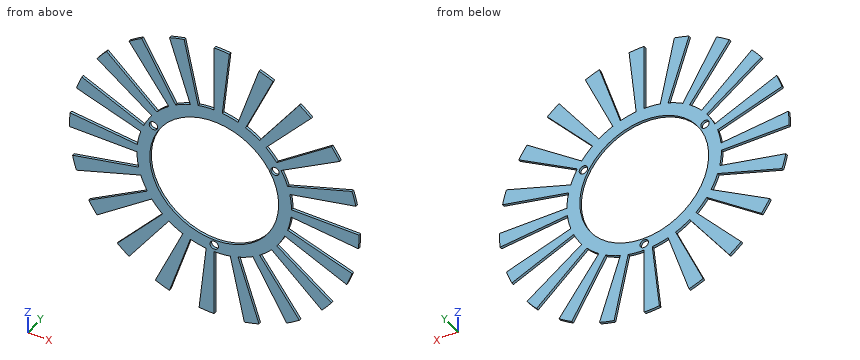
```python
from build123d import *

# Parameters (mm, degrees)
SKETCH1_R           = 30.25
SKETCH1_R_2         = 25.25
EXTRUDE_THIN1_DEPTH = 1
SKETCH2_R           = 1.65
CUT_EXTRUDE3_DEPTH  = 10
BOSS_EXTRUDE1_DEPTH = 1


with BuildPart() as part:
    # Sketch1 → Extrude-Thin1 (new body)
    with BuildSketch(Plane(origin=(0, 0, 0), x_dir=(1, 0, 0), z_dir=(0, 1, 0))):
        Circle(SKETCH1_R)
        Circle(SKETCH1_R_2, mode=Mode.SUBTRACT)
    extrude(amount=-EXTRUDE_THIN1_DEPTH)

    # Sketch2 → Cut-Extrude3 (cut)
    with BuildSketch(Plane(origin=(0, 0, 0), x_dir=(1, 0, 0), z_dir=(0, 1, 0))):
        with Locations((0, 27.5)):
            Circle(SKETCH2_R)
        with Locations((23.815698604, -13.75)):
            Circle(SKETCH2_R)
        with Locations((-23.815698604, -13.75)):
            Circle(SKETCH2_R)
    extrude(amount=-CUT_EXTRUDE3_DEPTH, mode=Mode.SUBTRACT)

    # Sketch5 → Boss-Extrude1 (add)
    with BuildSketch(Plane.XZ.offset(1)):
        with BuildLine():
            Line((0, 56.75), (0, 30.25))
            ThreePointArc((0, 30.25), (1.583162676, 30.208543426), (3.161986014, 30.084287335))
            Line((3.161986014, 30.084287335), (5.93199029, 56.439117562))
            ThreePointArc((5.93199029, 56.439117562), (2.970065517, 56.672226097), (0, 56.75))
        make_face()
        with BuildLine():
            Line((17.536714431, 53.9724573), (9.34776408, 28.769459618))
            ThreePointArc((9.34776408, 28.769459618), (10.840630474, 28.240807902), (12.303783453, 27.634750094))
            Line((12.303783453, 27.634750094), (23.082304495, 51.843704721))
            ThreePointArc((23.082304495, 51.843704721), (20.337381137, 52.980689204), (17.536714431, 53.9724573))
        make_face()
        with BuildLine():
            Line((33.356813068, 45.911714431), (17.780503882, 24.47276408))
            ThreePointArc((17.780503882, 24.47276408), (19.036941829, 23.508665334), (20.241200842, 22.480130971))
            Line((20.241200842, 22.480130971), (37.973161911, 42.173468846))
            ThreePointArc((37.973161911, 42.173468846), (35.713932192, 44.103033313), (33.356813068, 45.911714431))
        make_face()
        with BuildLine():
            Line((45.911714431, 33.356813068), (24.47276408, 17.780503882))
            ThreePointArc((24.47276408, 17.780503882), (25.36978468, 16.475330809), (26.197268464, 15.125))
            Line((26.197268464, 15.125), (49.146941665, 28.375))
            ThreePointArc((49.146941665, 28.375), (47.594554731, 30.908265237), (45.911714431, 33.356813068))
        make_face()
        with BuildLine():
            Line((53.9724573, 17.536714431), (28.769459618, 9.34776408))
            ThreePointArc((28.769459618, 9.34776408), (29.219256245, 7.829276114), (29.588964922, 6.289328647))
            Line((29.588964922, 6.289328647), (55.509876342, 11.798988454))
            ThreePointArc((55.509876342, 11.798988454), (54.816290642, 14.68798081), (53.9724573, 17.536714431))
        make_face()
        with BuildLine():
            Line((56.75, 0), (30.25, 0))
            ThreePointArc((30.25, 0), (30.208543426, -1.583162676), (30.084287335, -3.161986014))
            Line((30.084287335, -3.161986014), (56.439117562, -5.93199029))
            ThreePointArc((56.439117562, -5.93199029), (56.672226097, -2.970065517), (56.75, 0))
        make_face()
        with BuildLine():
            Line((53.9724573, -17.536714431), (28.769459618, -9.34776408))
            ThreePointArc((28.769459618, -9.34776408), (28.240807902, -10.840630474), (27.634750094, -12.303783453))
            Line((27.634750094, -12.303783453), (51.843704721, -23.082304495))
            ThreePointArc((51.843704721, -23.082304495), (52.980689204, -20.337381137), (53.9724573, -17.536714431))
        make_face()
        with BuildLine():
            Line((45.911714431, -33.356813068), (24.47276408, -17.780503882))
            ThreePointArc((24.47276408, -17.780503882), (23.508665334, -19.036941829), (22.480130971, -20.241200842))
            Line((22.480130971, -20.241200842), (42.173468846, -37.973161911))
            ThreePointArc((42.173468846, -37.973161911), (44.103033313, -35.713932192), (45.911714431, -33.356813068))
        make_face()
        with BuildLine():
            Line((33.356813068, -45.911714431), (17.780503882, -24.47276408))
            ThreePointArc((17.780503882, -24.47276408), (16.475330809, -25.36978468), (15.125, -26.197268464))
            Line((15.125, -26.197268464), (28.375, -49.146941665))
            ThreePointArc((28.375, -49.146941665), (30.908265237, -47.594554731), (33.356813068, -45.911714431))
        make_face()
        with BuildLine():
            Line((17.536714431, -53.9724573), (9.34776408, -28.769459618))
            ThreePointArc((9.34776408, -28.769459618), (7.829276114, -29.219256245), (6.289328647, -29.588964922))
            Line((6.289328647, -29.588964922), (11.798988454, -55.509876342))
            ThreePointArc((11.798988454, -55.509876342), (14.68798081, -54.816290642), (17.536714431, -53.9724573))
        make_face()
        with BuildLine():
            Line((0, -56.75), (0, -30.25))
            ThreePointArc((0, -30.25), (-1.583162676, -30.208543426), (-3.161986014, -30.084287335))
            Line((-3.161986014, -30.084287335), (-5.93199029, -56.439117562))
            ThreePointArc((-5.93199029, -56.439117562), (-2.970065517, -56.672226097), (0, -56.75))
        make_face()
        with BuildLine():
            Line((-17.536714431, -53.9724573), (-9.34776408, -28.769459618))
            ThreePointArc((-9.34776408, -28.769459618), (-10.840630474, -28.240807902), (-12.303783453, -27.634750094))
            Line((-12.303783453, -27.634750094), (-23.082304495, -51.843704721))
            ThreePointArc((-23.082304495, -51.843704721), (-20.337381137, -52.980689204), (-17.536714431, -53.9724573))
        make_face()
        with BuildLine():
            Line((-33.356813068, -45.911714431), (-17.780503882, -24.47276408))
            ThreePointArc((-17.780503882, -24.47276408), (-19.036941829, -23.508665334), (-20.241200842, -22.480130971))
            Line((-20.241200842, -22.480130971), (-37.973161911, -42.173468846))
            ThreePointArc((-37.973161911, -42.173468846), (-35.713932192, -44.103033313), (-33.356813068, -45.911714431))
        make_face()
        with BuildLine():
            Line((-45.911714431, -33.356813068), (-24.47276408, -17.780503882))
            ThreePointArc((-24.47276408, -17.780503882), (-25.36978468, -16.475330809), (-26.197268464, -15.125))
            Line((-26.197268464, -15.125), (-49.146941665, -28.375))
            ThreePointArc((-49.146941665, -28.375), (-47.594554731, -30.908265237), (-45.911714431, -33.356813068))
        make_face()
        with BuildLine():
            Line((-53.9724573, -17.536714431), (-28.769459618, -9.34776408))
            ThreePointArc((-28.769459618, -9.34776408), (-29.219256245, -7.829276114), (-29.588964922, -6.289328647))
            Line((-29.588964922, -6.289328647), (-55.509876342, -11.798988454))
            ThreePointArc((-55.509876342, -11.798988454), (-54.816290642, -14.68798081), (-53.9724573, -17.536714431))
        make_face()
        with BuildLine():
            Line((-56.75, 0), (-30.25, 0))
            ThreePointArc((-30.25, 0), (-30.208543426, 1.583162676), (-30.084287335, 3.161986014))
            Line((-30.084287335, 3.161986014), (-56.439117562, 5.93199029))
            ThreePointArc((-56.439117562, 5.93199029), (-56.672226097, 2.970065517), (-56.75, 0))
        make_face()
        with BuildLine():
            Line((-53.9724573, 17.536714431), (-28.769459618, 9.34776408))
            ThreePointArc((-28.769459618, 9.34776408), (-28.240807902, 10.840630474), (-27.634750094, 12.303783453))
            Line((-27.634750094, 12.303783453), (-51.843704721, 23.082304495))
            ThreePointArc((-51.843704721, 23.082304495), (-52.980689204, 20.337381137), (-53.9724573, 17.536714431))
        make_face()
        with BuildLine():
            Line((-45.911714431, 33.356813068), (-24.47276408, 17.780503882))
            ThreePointArc((-24.47276408, 17.780503882), (-23.508665334, 19.036941829), (-22.480130971, 20.241200842))
            Line((-22.480130971, 20.241200842), (-42.173468846, 37.973161911))
            ThreePointArc((-42.173468846, 37.973161911), (-44.103033313, 35.713932192), (-45.911714431, 33.356813068))
        make_face()
        with BuildLine():
            Line((-33.356813068, 45.911714431), (-17.780503882, 24.47276408))
            ThreePointArc((-17.780503882, 24.47276408), (-16.475330809, 25.36978468), (-15.125, 26.197268464))
            Line((-15.125, 26.197268464), (-28.375, 49.146941665))
            ThreePointArc((-28.375, 49.146941665), (-30.908265237, 47.594554731), (-33.356813068, 45.911714431))
        make_face()
        with BuildLine():
            Line((-17.536714431, 53.9724573), (-9.34776408, 28.769459618))
            ThreePointArc((-9.34776408, 28.769459618), (-7.829276114, 29.219256245), (-6.289328647, 29.588964922))
            Line((-6.289328647, 29.588964922), (-11.798988454, 55.509876342))
            ThreePointArc((-11.798988454, 55.509876342), (-14.68798081, 54.816290642), (-17.536714431, 53.9724573))
        make_face()
    extrude(amount=-BOSS_EXTRUDE1_DEPTH)


solid = part.part
```
Work out the finished part from the listing and answer in its coordinate system (mm). Give positions to 0.01 mm unless a question says otherwise; leave off trailing zeros. Loops run counter-clockwise (first coordinate to the right, second up) from the corner with the lowest first, then second, coordinate; pieces in that order, holes last. Notation, with made-up numbers: (89.5, 4) -> (132.5, 4) arc R14 ccw to (132.5, 13) -> close; hole circle Ø1 at (-2, 78.25). An arc over 180 degrees is marked (long way). Use CSV: the item, a comma, the result in double quotes.
1. The part is cut by section A-A (z = 44.5). Write down the section's boundary in (x, y).
Found:
outline,"(-32.33, -1) -> (-25.69, -1) -> (-25.69, 0) -> (-32.33, 0) -> close; (-14.46, -1) -> (-9.46, -1) -> (-9.46, 0) -> (-14.46, 0) -> close; (0, -1) -> (4.68, -1) -> (4.68, 0) -> (0, 0) -> close; (14.46, -1) -> (19.81, -1) -> (19.81, 0) -> (14.46, 0) -> close; (32.33, -1) -> (35.22, -1) -> (35.22, 0) -> (32.33, 0) -> close"
2. Flat-ended cylindrical pins translate along their axes: pin 1 Ø3 at (x, z) = (0, -27.5) entering from -Y; pin 2 Ø0.5 at (y, z) = (-0.5, -47) entering from +X. Find the tip coordinate at first contact, or state that the pin passes through.
Found:
pin 1,"through"
pin 2,"x = 32.17"
3. Straight lines are drawn through the part: line 1 (X direction, y = -0.15, z = 33.5); line 2 (X direction, y = -0.25, z = -27.5); line 3 (Z direction, x = 0.5, y = -0.7). For each, find the intervals that lie inside material, in ascending order.
Found:
line 1,"-45.81 to -37.21, -24.34 to -19.34, -10.88 to -7.12, 0 to 3.52, 10.88 to 14.92, 24.34 to 30.16"
line 2,"-47.63 to -37.85, -24.76 to -19.98, -12.6 to -1.65, 1.65 to 12.6, 15.88 to 19.98, 30.54 to 37.85"
line 3,"-30.25 to -29.07, -25.93 to -25.25, 25.25 to 56.75"
4. The part is cut by section C-C (z = 13.75). Write down the section's boundary in (x, y), then the cut area to 3 significant figures.
Found:
outline,"(-42.32, -1) -> (-30.88, -1) -> (-30.88, 0) -> (-42.32, 0) -> close; (-26.94, -1) -> (-25.47, -1) -> (-25.47, 0) -> (-26.94, 0) -> close; (-22.17, -1) -> (-21.18, -1) -> (-21.18, 0) -> (-22.17, 0) -> close; (21.18, -1) -> (22.17, -1) -> (22.17, 0) -> (21.18, 0) -> close; (25.47, -1) -> (26.94, -1) -> (26.94, 0) -> (25.47, 0) -> close; (42.32, -1) -> (55.06, -1) -> (55.06, 0) -> (42.32, 0) -> close"
area,"29.1 mm^2"
5. The part is cut by section B-B (y = -0.15). State how many separate pieces and enclosed holes the cut face has, then the cut area to 3 significant figures.
Found:
separate pieces,"1"
enclosed holes,"4"
area,"3,260 mm^2"
6. The part is cut by section D-D (x = 44.5). Write down the section's boundary in (y, z), then the cut area to 3 significant figures.
Found:
outline,"(-1, -35.22) -> (0, -35.22) -> (0, -32.33) -> (-1, -32.33) -> close; (-1, -19.81) -> (0, -19.81) -> (0, -14.46) -> (-1, -14.46) -> close; (-1, -4.68) -> (0, -4.68) -> (0, 0) -> (-1, 0) -> close; (-1, 9.46) -> (0, 9.46) -> (0, 14.46) -> (-1, 14.46) -> close; (-1, 25.69) -> (0, 25.69) -> (0, 32.33) -> (-1, 32.33) -> close"
area,"24.6 mm^2"
